from build123d import *

# Parameters (mm, degrees)
F3_DEPTH     = 10.0076
F4_DEPTH     = 40.005
F6_START     = -19.9898
F6_DEPTH     = 10.0076
F7_DEPTH     = 10.0076
F9_START     = 20.2438
F2_R         = 3.2004
F9_DEPTH     = 9.4996
F10_DEPTH    = 10.2616
F11_START    = 20.0152
F11_DEPTH    = 9.9822
F12_START    = -19.7612
F12_DEPTH    = 11.6078
F13_DEPTH    = 9.7536
F14_T1_DEPTH = 13.1863686745
F15_T1_DEPTH = 65.405
F16_R        = 2.54


# Not quite as in the source:
# - a fillet or chamfer that OpenCascade refuses, or shapes differently, is made with other operations: its cross-section is extruded or revolved along the edge and cut away or added


with BuildPart() as f3:
    # F0 (on Front) → F3 (new body)
    with BuildSketch(Plane.XZ):
        with BuildLine():
            ThreePointArc((-5.9119830007, 5.0038), (-3.8726462994, 1.4188735822), (0, 0))
            ThreePointArc((0, 0), (3.8726462994, 1.4188735822), (5.9119830007, 5.0038))
            ThreePointArc((5.9119830007, 5.0038), (5.9737602169, 5.4973887019), (5.9944, 5.9944))
            ThreePointArc((5.9944, 5.9944), (-0.4970112981, 11.9681602169), (-5.9119830007, 5.0038))
        make_face()
        with BuildLine():
            ThreePointArc((-0.3048, 3.0127385839), (0, 8.9916), (0.3048, 3.0127385839))
            Line((0.3048, 3.0127385839), (0.3048, 2.808547348))
            ThreePointArc((0.3048, 2.808547348), (0, 2.794), (-0.3048, 2.808547348))
            Line((-0.3048, 2.808547348), (-0.3048, 3.0127385839))
        make_face(mode=Mode.SUBTRACT)
        with BuildLine():
            Line((-19.9898, 0), (0, 0))
            ThreePointArc((0, 0), (-3.8726462994, 1.4188735822), (-5.9119830007, 5.0038))
            Line((-5.9119830007, 5.0038), (-19.9898, 5.0038))
            Line((-19.9898, 5.0038), (-19.9898, 0))
        make_face()
    extrude(amount=-F3_DEPTH)

    # F0 (on Front) → F4 (join)
    with BuildSketch(Plane.XZ):
        with BuildLine():
            Line((0.3048, 2.808547348), (0.3048, 3.0127385839))
            ThreePointArc((0.3048, 3.0127385839), (0, 8.9916), (-0.3048, 3.0127385839))
            Line((-0.3048, 3.0127385839), (-0.3048, 2.808547348))
            ThreePointArc((-0.3048, 2.808547348), (0, 2.794), (0.3048, 2.808547348))
        make_face()
    extrude(amount=-F4_DEPTH)

    # F0 (on Front) → F6 (join)
    with BuildSketch(Plane.XZ.offset(F6_START)):
        with BuildLine():
            ThreePointArc((-5.9119830007, 5.0038), (-3.8726462994, 1.4188735822), (0, 0))
            ThreePointArc((0, 0), (3.8726462994, 1.4188735822), (5.9119830007, 5.0038))
            ThreePointArc((5.9119830007, 5.0038), (5.9737602169, 5.4973887019), (5.9944, 5.9944))
            ThreePointArc((5.9944, 5.9944), (-0.4970112981, 11.9681602169), (-5.9119830007, 5.0038))
        make_face()
        with BuildLine():
            ThreePointArc((-0.3048, 3.0127385839), (0, 8.9916), (0.3048, 3.0127385839))
            Line((0.3048, 3.0127385839), (0.3048, 2.808547348))
            ThreePointArc((0.3048, 2.808547348), (0, 2.794), (-0.3048, 2.808547348))
            Line((-0.3048, 2.808547348), (-0.3048, 3.0127385839))
        make_face(mode=Mode.SUBTRACT)
        with BuildLine():
            Line((-19.9898, 0), (0, 0))
            ThreePointArc((0, 0), (-3.8726462994, 1.4188735822), (-5.9119830007, 5.0038))
            Line((-5.9119830007, 5.0038), (-19.9898, 5.0038))
            Line((-19.9898, 5.0038), (-19.9898, 0))
        make_face()
    extrude(amount=-F6_DEPTH)

    # F2 (on offset) → F7 (join)
    with BuildSketch(Plane.XZ.offset(-40.005)):
        with BuildLine():
            ThreePointArc((-1.5118372742, 0.1937811178), (-4.4229342387, 1.9483545134), (-5.9119830007, 5.0038))
            Line((-5.9119830007, 5.0038), (-19.9898, 5.0038))
            Line((-19.9898, 5.0038), (-19.9898, 0))
            Line((-19.9898, 0), (-1.5366753453, 0))
            ThreePointArc((-1.5366753453, 0), (-1.4389921182, 0.0859617436), (-1.5118372742, 0.1937811178))
        make_face()
    extrude(amount=F7_DEPTH)

    # F2 (on offset) → F9 (join)
    with BuildSketch(Plane.XZ.offset(-40.005).offset(F9_START)):
        with BuildLine():
            Line((0, 0.3048), (0, 0))
            ThreePointArc((0, 0), (3.8726462994, 1.4188735822), (5.9119830007, 5.0038))
            Line((5.9119830007, 5.0038), (5.6027011164, 5.0038))
            ThreePointArc((5.6027011164, 5.0038), (-3.6561886166, 10.353738592), (0, 0.3048))
        make_face()
        with Locations((0, 5.9944)):
            Circle(F2_R, mode=Mode.SUBTRACT)
        with BuildLine():
            ThreePointArc((5.9119830007, 5.0038), (3.8726462994, 1.4188735822), (0, 0))
            Line((0, 0), (19.9898, 0))
            Line((19.9898, 0), (19.9898, 5.0038))
            Line((19.9898, 5.0038), (5.9119830007, 5.0038))
        make_face()
    extrude(amount=F9_DEPTH)

    # F0 (on Front) → F10 (join)
    with BuildSketch(Plane.XZ):
        with BuildLine():
            ThreePointArc((6.2722573002, 5.0038), (4.8747199854, 1.9250505355), (2.0951536077, 0))
            Line((2.0951536077, 0), (19.9898, 0))
            Line((19.9898, 0), (19.9898, 5.0038))
            Line((19.9898, 5.0038), (6.2722573002, 5.0038))
        make_face()
    extrude(amount=-F10_DEPTH)

    # F2 (on offset) → F11 (join)
    with BuildSketch(Plane.XZ.offset(-40.005).offset(F11_START)):
        with BuildLine():
            ThreePointArc((-1.5118372742, 0.1937811178), (-4.4229342387, 1.9483545134), (-5.9119830007, 5.0038))
            Line((-5.9119830007, 5.0038), (-19.9898, 5.0038))
            Line((-19.9898, 5.0038), (-19.9898, 0))
            Line((-19.9898, 0), (-1.5366753453, 0))
            ThreePointArc((-1.5366753453, 0), (-1.4389921182, 0.0859617436), (-1.5118372742, 0.1937811178))
        make_face()
    extrude(amount=F11_DEPTH)

    # F0 (on Front) → F12 (join)
    with BuildSketch(Plane.XZ.offset(F12_START)):
        with BuildLine():
            ThreePointArc((6.2722573002, 5.0038), (4.8747199854, 1.9250505355), (2.0951536077, 0))
            Line((2.0951536077, 0), (19.9898, 0))
            Line((19.9898, 0), (19.9898, 5.0038))
            Line((19.9898, 5.0038), (6.2722573002, 5.0038))
        make_face()
    extrude(amount=-F12_DEPTH)

    # F2 (on offset) → F13 (join)
    with BuildSketch(Plane.XZ.offset(-40.005)):
        with BuildLine():
            ThreePointArc((5.9119830007, 5.0038), (3.8726462994, 1.4188735822), (0, 0))
            Line((0, 0), (19.9898, 0))
            Line((19.9898, 0), (19.9898, 5.0038))
            Line((19.9898, 5.0038), (5.9119830007, 5.0038))
        make_face()
        with BuildLine():
            Line((0, 0.3048), (0, 0))
            ThreePointArc((0, 0), (3.8726462994, 1.4188735822), (5.9119830007, 5.0038))
            Line((5.9119830007, 5.0038), (5.6027011164, 5.0038))
            ThreePointArc((5.6027011164, 5.0038), (-3.6561886166, 10.353738592), (0, 0.3048))
        make_face()
        with Locations((0, 5.9944)):
            Circle(F2_R, mode=Mode.SUBTRACT)
    extrude(amount=F13_DEPTH)

    # F14: fillet of radius 0.254 on 1 edges, made by hand

    # F14_s2 → F14_t1 (cut)
    with BuildSketch(Plane.XZ.offset(-10.2616)):
        with BuildLine():
            ThreePointArc((3.1394818053, 0.4747846154), (3.0195052872, 0.1890511444), (3.2650610775, 0))
            Line((3.2650610775, 0), (2.0951536077, 0))
            ThreePointArc((2.0951536077, 0), (2.628061469, 0.2137605098), (3.1394818053, 0.4747846154))
        make_face()
    extrude(amount=F14_T1_DEPTH, mode=Mode.SUBTRACT)

    # F15: fillet of radius 5.08 on 2 edges, made by hand

    # F15_s2 → F15_t1 (cut)
    with BuildSketch(Plane.XZ.offset(-52.705)):
        with BuildLine():
            ThreePointArc((-14.9098, 5.0038), (-18.5019024484, 3.5159024484), (-19.9898, -0.0762))
            Line((-19.9898, -0.0762), (-19.9898, 5.0038))
            Line((-19.9898, 5.0038), (-14.9098, 5.0038))
        make_face()
        with BuildLine():
            ThreePointArc((19.9898, -0.0762), (18.5019024484, 3.5159024484), (14.9098, 5.0038))
            Line((14.9098, 5.0038), (19.9898, 5.0038))
            Line((19.9898, 5.0038), (19.9898, -0.0762))
        make_face()
    extrude(amount=F15_T1_DEPTH, mode=Mode.SUBTRACT)

    # F16
    f16_edges = [f3.edges().sort_by_distance(p)[0] for p in [
        (10.256251, 40.005, 5.0038),
        (-10.410892, 40.005, 5.0038),
        (-10.410892, 0, 5.0038),
        (10.591029, 0, 5.0038),
        (-18.47486, 0, 3.542743),
        (-18.47486, 40.005, 3.542743),
        (18.47486, 40.005, 3.542743),
        (18.47486, 0, 3.542743),
    ]]
    fillet(f16_edges, radius=F16_R)


solid = f3.part
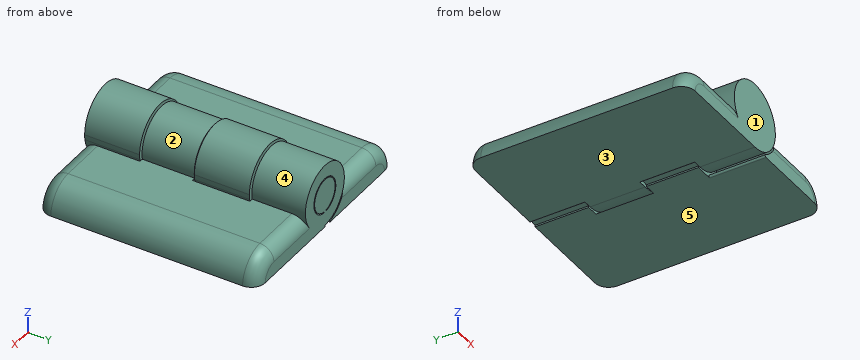
The model under review builds one solid part; all positions refer to its coordinate system, in mm. Face numbers are marked on the shaded views. A direction names the side the tool comes from. Round coordinates to 2 decimals unless told otherwise and drop trailing zeros. Loops run counter-clockwise (first coordinate to the right, second up) from the corner with the lowest first, then second, coordinate; pieces in that order, holes last. Notation, with made-up numbers: (45, -1) -> (87, -1) arc R17 ccw to (87, 4) -> close; hole circle Ø7 at (48.5, 46). An arc over 180 degrees is marked (long way). Return JSON: item names as keys, results as strings.
(1) Add section D-D on x = -9. Write out the cut boundary in (y, z) (3 decimals).
Solved:
{"outline": "(0, 0) -> (40.005, 0) -> (40.005, 2.464) arc R2.54 ccw to (37.465, 5.004) -> (2.54, 5.004) arc R2.54 ccw to (0, 2.464) -> close"}
(2) The part is to be moulded in two halves that separate along Z. For the marked faces 1, 2 and 3, say which applies: released by +Z, released by -Z, zero draft, split by the parting line, or undercut.
Solved:
{"face 1": "zero draft", "face 2": "undercut", "face 3": "released by -Z"}
(3) Add section B-B on x = 1. State how many separate pieces and enclosed holes the cut face has, plus the area to 3 significant figures.
Solved:
{"separate pieces": "5", "enclosed holes": "0", "area": "456 mm2"}
(4) For line 1 (Y direction, x = -4.5, z = 6.5) (3 decimals); line 2 (Z direction, x = -2, y = 30.5); line 3 (X direction, y = 17, z = 7.5), list the stretches that pass through material, from the lowest coordinate up.
Solved:
{"line 1": "0 to 10.008, 10.262 to 19.761, 19.99 to 29.997, 30.251 to 40.005", "line 2": "0 to 0.34, 0.67 to 3.5, 3.76 to 8.23, 8.49 to 11.32", "line 3": "-5.49 to -2.82, -2.59 to 2.59, 2.82 to 5.49"}
(5) Add section C-C on z = 11. Write out the cut boundary in (x, y) (3 decimals).
Solved:
{"outline": "(-3.298, 0) -> (3.298, 0) -> (3.298, 10.008) -> (-3.298, 10.008) -> close; (-3.298, 19.99) -> (3.298, 19.99) -> (3.298, 29.997) -> (-3.298, 29.997) -> close; (-2.705, 10.262) -> (2.705, 10.262) -> (2.705, 19.761) -> (-2.705, 19.761) -> close; (-2.705, 30.251) -> (2.705, 30.251) -> (2.705, 40.005) -> (-2.705, 40.005) -> close"}
(6) For pin 1 (12 mm diameter, centred on x = 15, y = 6, fed in from +Z); pin 2 (5 mm diameter, centred on x = -10.5, z = 6, fed in from -Y); pin 3 (6 mm diameter, centred on y = 13, z = 8.5, fed in from +X), all flat-tipped, find the tip position at first contact; note any pin that passes through.
Solved:
{"pin 1": "z = 5", "pin 2": "y = 0.22", "pin 3": "x = 5.69"}
(7) For the marked faces 4 and 5, list the 3-axis set-ups (+Z, -Z, +X, -X, +Y, -Y) from which the entire face can be reached by the end or side of a thin tool; tool diameter is ignored.
Solved:
{"face 4": "+Y", "face 5": "-Z, +X, -X, +Y, -Y"}
(8) Add section A-A on y = 17. Write out the cut boundary in (x, z).
Solved:
{"outline": "(-19.99, 0) -> (-1.54, 0) arc R0.1 ccw to (-1.51, 0.19) arc R5.99 cw to (-5.91, 5) -> (-14.91, 5) arc R5.08 ccw to start; (0, 0) -> (19.99, 0) arc R5.08 ccw to (14.91, 5) -> (5.6, 5) arc R5.69 ccw (long way) to (0, 0.3) -> close; hole (-0.3, 2.81) -> (-0.3, 3.01) arc R3 cw (long way) to (0.3, 3.01) -> (0.3, 2.81) arc R3.2 ccw (long way) to start"}
